Autodesk Fusion 360 part; units mm, degrees
sketch "スケッチ1" plane through (0, 0, 0) normal (0, 0, 1) x (1, 0, 0)
  line L0 (2.5, 186) -> (-92.5, 186)
  line L1 (-92.5, 186) -> (-92.5, -186)
  line L2 (-92.5, -186) -> (2.5, -186)
  line L3 (92.5, -100) -> (92.5, 180)
  line L4 (89.5161, 180) -> (-92.5, -186) construction
  line L5 (-92.5, 186) -> (63.5083, -127.7032) construction
  line L6 (2.5, 186) -> (2.5, 180)
  line L7 (2.5, 180) -> (92.5, 180)
  line L8 (-92.5, -186) -> (2.5, -186) construction
  line L9 (92.5, -100) -> (2.5, -186)
  dimension "d2" = 372
  dimension "d5" = 95
extrude "押し出し1" add sketch "スケッチ1" along normal blind 8
chamfer "面取り1" distance 30 angle 45 2 edges at (-92.5, -186, 4) (-92.5, 186, 4)
sketch "スケッチ2" plane through (0, 0, 8) normal (0, 0, 1) x (-1, 0, 0)
  line L0 (62.5, -186) -> (92.5, -156)
  line L1 (92.5, -156) -> (92.5, 156)
  line L2 (92.5, 156) -> (62.5, 186)
  line L3 (62.5, 186) -> (-2.5, 186)
  line L4 (-2.5, 186) -> (-92.5, 100)
  line L5 (-92.5, 100) -> (-92.5, -180)
  line L6 (-92.5, -180) -> (-2.5, -180)
  line L7 (-2.5, -180) -> (-2.5, -186)
  line L8 (-2.5, -186) -> (62.5, -186)
  line L9 (-92.5, -180) -> (-52.5, -180) construction
  line L10 (-52.5, -180) -> (-52.5, -120) construction
  line L11 (-52.5, -120) -> (-92.5, -120) construction
  line L12 (-92.5, -120) -> (-92.5, -180) construction
  line L13 (-52.5, -120) -> (-52.5, -50) construction
  line L14 (-52.5, -50) -> (-52.5, 20) construction
  point P0 (-52.5, -120)
  point P1 (-52.5, -50)
  point P2 (-52.5, 20)
  dimension "d10" = 40
  dimension "d11" = 60
  dimension "d12" = 70
  dimension "d13" = 70
hole "穴1" at (52.5, 120, 8) at (52.5, 50, 8) at (52.5, -20, 8) direction (0, 0, -1) diameter 22 end through all
equation "d5 = 30 mm + 65 mm"
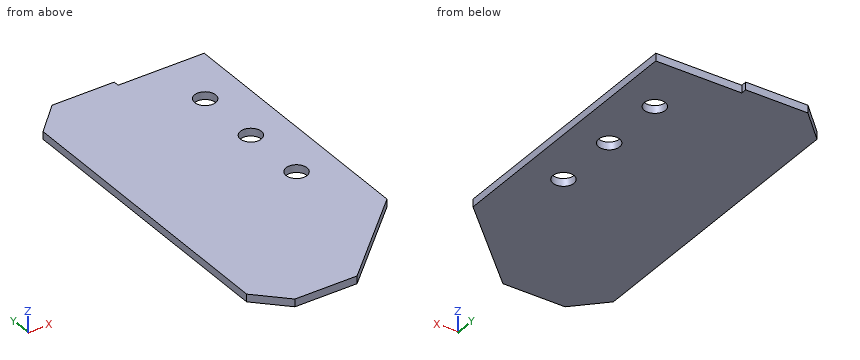
Check sheet for the modelled part. Datum: model origin and axes. Units: mm. Coordinates: 2 decimals unless noted, no trailing zeros. Write each loop counter-clockwise with the first axis right and the second up, starting at its lowest first coordinate (ties: lowest second). Pieces come first, ordered by that corner, then holes. Notation, with made-up numbers: M 13,45 L 28,45 A27 ccw 28,77 Z; hole C 20,-8.75 d9. An arc over 180 degrees is marked long. Write item = value, one per line. Start each with the question number.
1. Sectioned sample at B-B (z = 6.5). Record the cut outline in (x, y), then the cut area to 3 significant figures.
2. Sectioned sample at D-D (y = 127.5). Record the cut outline in (x, z).
3. Sectioned sample at A-A (y = 50). Record the cut outline in (x, z), then the cut area to 3 significant figures.
4. Thickness scan on probe 1 along X at (y, z) = (120, 3.5); probe 2 along Y at (x, z) = (52.5, 2); probe 3 along X at (y, z) = (53.5, 5.5). Record the ranges inside material, lowest first.
5. Go/stop test with flat-tipped pins: pin 1 (3 mm diameter, centred on x = 67.5, z = 2.5, fed in from +Y); pin 2 (3 mm diameter, centred on x = 1.5, y = -40.5, fed in from -Z). Record where each tip stops, or that it passes through.
6. Sectioned sample at C-C (x = 52.5). Record the cut outline in (y, z).
The answers:
q1.outline = M -92.5,-156 L -62.5,-186 L 2.5,-186 L 92.5,-100 L 92.5,180 L 2.5,180 L 2.5,186 L -62.5,186 L -92.5,156 Z; hole C 52.5,-20 d22; hole C 52.5,50 d22; hole C 52.5,120 d22
q1.area = 62,400 mm²
q2.outline = M -92.5,0 L 44.45,0 L 44.45,8 L -92.5,8 Z; M 60.55,0 L 92.5,0 L 92.5,8 L 60.55,8 Z
q3.outline = M -92.5,0 L 41.5,0 L 41.5,8 L -92.5,8 Z; M 63.5,0 L 92.5,0 L 92.5,8 L 63.5,8 Z
q3.area = 1,300 mm²
q4.probe_1 = -92.5 to 41.5, 63.5 to 92.5
q4.probe_2 = -138.22 to -31, -9 to 39, 61 to 109, 131 to 180
q4.probe_3 = -92.5 to 42.07, 62.93 to 92.5
q5.pin_1 = 180
q5.pin_2 = 0
q6.outline = M -138.22,0 L -31,0 L -31,8 L -138.22,8 Z; M -9,0 L 39,0 L 39,8 L -9,8 Z; M 61,0 L 109,0 L 109,8 L 61,8 Z; M 131,0 L 180,0 L 180,8 L 131,8 Z
